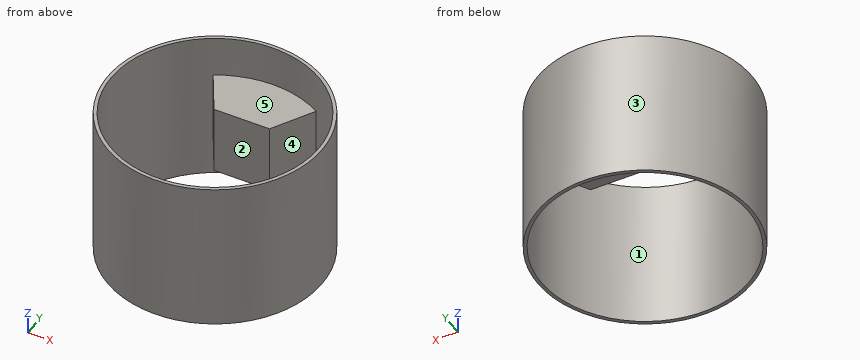
```python
from build123d import *

# Parameters (mm, degrees)
SKETCH_1_R      = 155
SKETCH_1_R_2    = 150
EXTRUDE_1_DEPTH = 110
EXTRUDE_2_DEPTH = 50


with BuildPart() as part:
    # 草图1 → 凸台-拉伸1 (new body, symmetric)
    with BuildSketch(Plane.XY):
        Circle(SKETCH_1_R)
        Circle(SKETCH_1_R_2, mode=Mode.SUBTRACT)
    extrude(amount=EXTRUDE_1_DEPTH, both=True)

    # 草图2 → 凸台-拉伸2 (add, symmetric)
    with BuildSketch(Plane.XY):
        with BuildLine():
            Line((-40.414518843, 70), (-75, 129.903810568))
            ThreePointArc((-75, 129.903810568), (0, 150), (75, 129.903810568))
            Line((75, 129.903810568), (40.414518843, 70))
            Line((40.414518843, 70), (-40.414518843, 70))
        make_face()
    extrude(amount=EXTRUDE_2_DEPTH, both=True)


solid = part.part
```
For this review, take the finished solid that the model builds, in its own axes (mm). Face numbers are marked on the shaded views. A direction names the side the tool comes from. Coordinates: 2 decimals unless noted, no trailing zeros. Order: outer loops, then holes, each group sorted by start corner. A loop starts at its lowest first (then second) coordinate and runs counter-clockwise, first axis right, second up. Notation, with made-up numbers: (46.25, 49.5) - (80.25, 49.5) arc R35 ccw to (80.25, 81.5) - close; hole circle Ø9 at (-31, -38). An arc over 180 degrees is marked (long way). Answer as a JSON object with one key per item and string values. Group by question number.
1. We need section C-C on z = 24. State the section outline as (x, y) points.
2. We need section A-A on x = 0. State the section outline as (y, z) points.
3. The part is to be moulded in two halves that separate along Y. For the marked faces 1, 2 and 3, say which applies: pulls with the +Y half, pulls with the -Y half, needs draft (parallel to the pull), parting line crosses it, or undercut.
4. Clearance check with flat-ended pins moving along their axes: P1, Ø1.5, axis at x = -41.5, z = 16.5, coming from the -Y side; P2, Ø2, axis at x = -70, z = -3.5, coming from the -Y side; P3, Ø8, axis at x = -92, z = -43, coming from the +Y side. State where each tip first meets the part, or that it passes through.
5. We need section B-B on y = -34. State the section outline as (x, z) points (3 decimals).
6. For probe 1 along Y at (x, z) = (0, -27); probe 2 along X at (y, z) = (96, 33.5); probe 3 along X at (y, z) = (-34, 75) (3 decimals), list the stretches that pass through material, from the lowest coordinate up.
7. For the marked faces 4 and 5, list the 3-axis set-ups (+Z, -Z, +X, -X, +Y, -Y) from which the entire face can be reached by the end or side of a thin tool; tool diameter is ignored.
8. We need section D-D on y = 0. State the section outline as (x, z) points.
Final values:
{
 "1": {"outline": "circle Ø310 at (0, 0); hole (-75, 129.9) arc R150 ccw (long way) to (75, 129.9) - (40.41, 70) - (-40.41, 70) - close"},
 "2": {"outline": "(-155, -110) - (-150, -110) - (-150, 110) - (-155, 110) - close; (70, -50) - (150, -50) - (150, -110) - (155, -110) - (155, 110) - (150, 110) - (150, 50) - (70, 50) - close"},
 "3": {"face 1": "undercut", "face 2": "undercut", "face 3": "parting line crosses it"},
 "4": {"P1": "y = -149.55", "P2": "y = -138.79", "P3": "y = 127.6"},
 "5": {"outline": "(-151.225, -110) - (-146.096, -110) - (-146.096, 110) - (-151.225, 110) - close; (146.096, -110) - (151.225, -110) - (151.225, 110) - (146.096, 110) - close"},
 "6": {"probe 1": "-155 to -150, 70 to 155", "probe 2": "-121.69 to -115.26, -55.43 to 55.43, 115.26 to 121.69", "probe 3": "-151.225 to -146.096, 146.096 to 151.225"},
 "7": {"face 4": "+Z, -Z", "face 5": "+Z"},
 "8": {"outline": "(-155, -110) - (-150, -110) - (-150, 110) - (-155, 110) - close; (150, -110) - (155, -110) - (155, 110) - (150, 110) - close"}
}
